Autodesk Inventor part; units mm, degrees
ref_plane "YZ Plane" through (0, 0, 0) normal (1, 0, 0) x (0, 1, 0)
ref_plane "XZ Plane" through (0, 0, 0) normal (0, 1, 0) x (-1, 0, 0)
ref_plane "XY Plane" through (0, 0, 0) normal (0, 0, 1) x (1, 0, 0)
sketch "Sketch1" plane through (0, 0, 0) normal (0, 0, 1) x (1, 0, 0)
  line L0 (0, 0) -> (28.5, 0) construction
  line L1 (28.5, 0) -> (28.5, 27)
  line L2 (0, 0) -> (19, 0) construction
  line L3 (19, 0) -> (22, 0) construction
  line L4 (28.5, 0) -> (22, 0)
  line L5 (19, 0) -> (19, 2) construction
  line L6 (19, 2) -> (22, 0)
  line L7 (19, 2) -> (19, 21)
  line L8 (19, 21) -> (16, 21) construction
  line L9 (16, 21) -> (16, 23) construction
  line L10 (16, 23) -> (19, 21)
  line L11 (16, 23) -> (16, 26)
  line L12 (16, 26) -> (20, 26)
  line L13 (20, 26) -> (20, 29)
  line L14 (20, 29) -> (25.5, 29)
  line L15 (25.5, 29) -> (25.5, 39)
  line L16 (25.5, 39) -> (28.5, 39)
  line L17 (28.5, 39) -> (28.5, 33)
  line L18 (28.5, 33) -> (33.5, 33)
  line L19 (33.5, 33) -> (33.5, 36)
  line L20 (28.5, 27) -> (37, 27)
  line L21 (37, 27) -> (37, 36)
  line L22 (37, 36) -> (33.5, 36)
  line L23 (0, 0) -> (0, 8.384) construction
  dimension "d0" = 28.5
  dimension "d1" = 27
  dimension "d2" = 19
  dimension "d3" = 3
  dimension "d4" = 2
  dimension "d5" = 21
  dimension "d6" = 3
  dimension "d7" = 2
  dimension "d8" = 3
  dimension "d17" = 3
  dimension "d18" = 5.5
  dimension "d19" = 4
  dimension "d20" = 10
  dimension "d21" = 3
  dimension "d22" = 6
  dimension "d23" = 5
  dimension "d24" = 3
  dimension "d25" = 8.5
revolve "Revolution1" add sketch "Sketch1" angle 360 about axis through (0, 0, 0) along (0, 1, 0)
properties part number "Body Cap Base Feature" material "Bronze, Soft Tin"
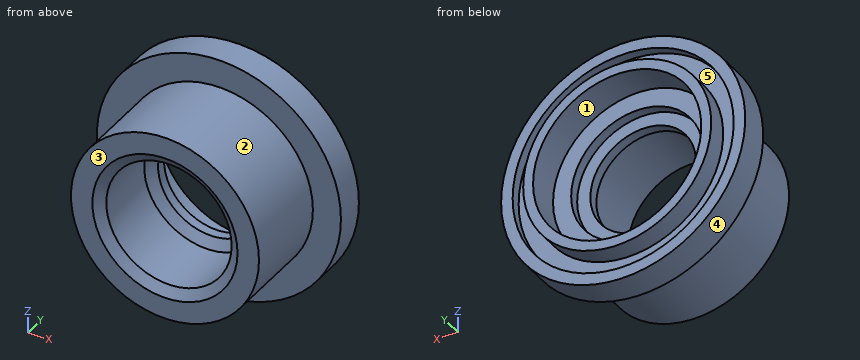
Design review of the part built by this model. Coordinates are the model's own, in mm. Face numbers are marked on the shaded views. A direction names the side the tool comes from. Coordinates: 2 decimals unless noted, no trailing zeros. Loops run counter-clockwise (first coordinate to the right, second up) from the corner with the lowest first, then second, coordinate; pieces in that order, holes last. Notation, with made-up numbers: (-37, 10.5) -> (-23, 10.5) arc R25 cw to (-23, 37.5) -> close; hole circle Ø11 at (48, -30). An arc over 180 degrees is marked (long way). Answer as a JSON object with one key per item and string values.
Q1. To check wall thickness, follow L1, parallel to X at y = 33.7, z = 0; L2, parallel to X at y = 10.75, z = 0; L3, parallel to Z at x = 0, y = 24.8. State the ranges of each line that lie inside material, in increasing order.
Answer block:
{"L1": "x = -37 to -33.5, -28.5 to -25.5, 25.5 to 28.5, 33.5 to 37", "L2": "x = -28.5 to -19, 19 to 28.5", "L3": "z = -28.5 to -16, 16 to 28.5"}
Q2. Tool access review of the marked faces 1 and 2: name each direction out of +Z, -Z, +X, -X, +Y, -Y from which nothing blocks a thin tool from reaching the whole face with its end or side.
Answer block:
{"face 1": "+Y", "face 2": "-Y"}
Q3. Take a section at D-D on z = 31.5. Give the boundary of the cut face in (x, y).
Answer block:
{"outline": "(-19.41, 27) -> (19.41, 27) -> (19.41, 36) -> (11.4, 36) -> (11.4, 33) -> (-11.4, 33) -> (-11.4, 36) -> (-19.41, 36) -> close"}
Q4. Clearance check with flat-ended pins moving along their axes: pin 1 Ø12 at (x, z) = (4, 6.5) entering from +Y; pin 2 Ø8 at (x, y) = (-10.5, 19.5) entering from +Z; pin 3 Ø2 at (x, z) = (17.5, -26.5) entering from -Y; pin 4 Ø3 at (x, z) = (-22.5, 1) entering from +Y. State where each tip first meets the part, or that it passes through.
Answer block:
{"pin 1": "passes through", "pin 2": "stops at z = 27.75", "pin 3": "stops at y = 27", "pin 4": "stops at y = 29"}
Q5. The part is to be moulded in two halves that separate along Z. For the marked faces 3, 4 and 5, say which applies: +Z half, -Z half, draft (parallel to the pull), parting line (faces both ways), or undercut.
Answer block:
{"face 3": "draft", "face 4": "parting line", "face 5": "undercut"}
Q6. Take a section at C-C on y = 32. Give the boundary of the cut face in (x, z).
Answer block:
{"outline": "circle Ø74 at (0, 0); hole circle Ø51 at (0, 0)"}
